```python
from build123d import *

# Parameters (mm, degrees)
SKETCH2_W           = 5
SKETCH2_H           = 21
SKETCH2_W_2         = 5.4
SKETCH2_H_2         = 20
BOSS_EXTRUDE1_DEPTH = 20
CIRPATTERN1_COUNT   = 16
SKETCH6_W           = 4
SKETCH6_H           = 4
CUT_EXTRUDE1_DEPTH  = 56.072679252
CHAMFER1_SIZE       = 1


with BuildPart() as part:
    # Sketch2 → Revolve1 (revolve)
    with BuildSketch(Plane.XY, mode=Mode.PRIVATE) as revolve1_sk:
        with Locations((17.5, 30.5)):
            Rectangle(SKETCH2_W, SKETCH2_H)
        with Locations((17.7, 10)):
            Rectangle(SKETCH2_W_2, SKETCH2_H_2)
    revolve(revolve1_sk.sketch.rotate(Axis((0, 0, 0), (0, 1, 0)), 90), axis=Axis((0, 0, 0), (0, 1, 0)))

    # Sketch4 → Boss-Extrude1 (add)
    with BuildSketch(Plane(origin=(0, 20, 0), x_dir=(1, 0, 0), z_dir=(0, 1, 0))):
        with BuildLine():
            ThreePointArc((-2.75, 20.213794795), (-1.37814843, 20.353395464), (0, 20.4))
            Line((0, 20.4), (0, 26))
            ThreePointArc((0, 26), (-0.62518076, 25.992482548), (-1.25, 25.96993454))
            ThreePointArc((-1.25, 25.96993454), (-2.215194302, 23.147942432), (-2.75, 20.213794795))
        make_face()
        with BuildLine():
            Line((0, 26), (0, 20.4))
            ThreePointArc((0, 20.4), (1.37814843, 20.353395464), (2.75, 20.213794795))
            ThreePointArc((2.75, 20.213794795), (2.215194302, 23.147942432), (1.25, 25.96993454))
            ThreePointArc((1.25, 25.96993454), (0.62518076, 25.992482548), (0, 26))
        make_face()
    boss_extrude1 = extrude(amount=-BOSS_EXTRUDE1_DEPTH)

    # CirPattern1: Boss-Extrude1 ×16 about axis
    cirpattern1_axis = Axis((0, 0, 0), (0, 1, 0))
    for i in range(1, CIRPATTERN1_COUNT):
        add(boss_extrude1.rotate(cirpattern1_axis, i * 360 / CIRPATTERN1_COUNT))

    # Sketch6 → Cut-Extrude1 (cut, through all)
    with BuildSketch(Plane(origin=(0, 41, 0), x_dir=(1, 0, 0), z_dir=(0, 1, 0))):
        with Locations((0, 15)):
            Rectangle(SKETCH6_W, SKETCH6_H)
    extrude(amount=-CUT_EXTRUDE1_DEPTH, mode=Mode.SUBTRACT)

    # Chamfer1
    chamfer1_edges = [part.edges().sort_by_distance(p)[0] for p in [
        (0, 41, 20),
    ]]
    chamfer(chamfer1_edges, length=CHAMFER1_SIZE)


solid = part.part
```
Check sheet for the modelled part. Datum: model origin and axes. Units: mm. A direction names the side the tool comes from. Coordinates: 2 decimals unless noted, no trailing zeros. Write each loop counter-clockwise with the first axis right and the second up, starting at its lowest first coordinate (ties: lowest second). Pieces come first, ordered by that corner, then holes. Notation, with made-up numbers: M 78.25,-14.5 L 94.25,-14.5 A16 ccw 94.25,11.5 Z; hole C 2,75.25 d1. An arc over 180 degrees is marked long. Write item = value, one per line. Start each with the question number.
1. Sectioned sample at A-A (y = 33). Record the cut outline in (x, z).
2. Thickness scan on probe 1 along Z at (x, y) = (0, 14.5); probe 2 along X at (y, z) = (3, 23); probe 3 along Z at (x, y) = (-22.5, 8). Record the ranges inside material, lowest first.
3. Mould release check, pull along Z, two halves, no side actions. Record for faces 5 (the cylindrical face through (14.766, 10.14, 17.913)), 6 (the cylindrical face through (-22.27, 10.14, -6.84)), 7 (the cylindrical face through (10.9, 10.1, -20.5)), 8 (the flat face through (6, 41, 14)): pulls with the +Z half, pulls with the -Z half, needs draft (parallel to the pull), parting line crosses it, or undercut.
4. Go/stop test with flat-tipped pins: pin 1 (1.5 mm diameter, centred on x = 12, z = 11.5, fed in from -Y); pin 2 (2.5 mm diameter, centred on y = 14.5, z = -15.5, fed in from -X); pin 3 (2.5 mm diameter, centred on y = 25, z = -16, fed in from +X); pin 4 (3 mm diameter, centred on x = 3, y = 26, fed in from -Z). Record where each tip stops, or that it passes through.
5. Tool access check on faces 1 (the cylindrical face through (-2.2, 10.1, -23.2)), 2 (the cylindrical face through (-17.956, 10.14, -14.838)), 3 (the flat face through (-8, 0, -14)), 4 (the cylindrical face through (11.35, 10.14, -16.95)). Record the directions out of +Z, -Z, +X, -X, +Y, -Y that give a thin tool (end or side, any length) a straight path to the whole face; none if there is none.
The answers:
q1.outline = C 0,0 d40; hole M -2,-17 L 2,-17 L 2,-14.87 A15 ccw long -2,-14.87 Z
q2.probe_1 = -26 to -17, 15 to 26
q2.probe_2 = -11.09 to -7.42, -2.25 to 2.25, 7.42 to 11.09
q2.probe_3 = -11.08 to -7.02, -2.37 to 2.37, 7.02 to 11.08
q3.face_5 = pulls with the +Z half
q3.face_6 = undercut
q3.face_7 = undercut
q3.face_8 = needs draft
q4.pin_1 = 0
q4.pin_2 = -18.94
q4.pin_3 = 13.51
q4.pin_4 = -19.94
q5.face_1 = -Z, +Y, -Y
q5.face_2 = -X, +Y, -Y
q5.face_3 = +Z, -Z, +X, -X, -Y
q5.face_4 = +Y, -Y
